from build123d import *

# Parameters (mm, degrees)
SKETCH1_W             = 60.96
SKETCH1_H             = 73.66
BOSS_EXTRUDE1_DEPTH   = 3.0734
FILLET1_R             = 2.54
F_8_CLEARANCE_HOLE1_D = 4.4958


with BuildPart() as part:
    # Sketch1 → Boss-Extrude1 (new body)
    with BuildSketch(Plane(origin=(0, 0, 0), x_dir=(1, 0, 0), z_dir=(0, 1, 0))):
        with Locations((30.48, 36.83)):
            Rectangle(SKETCH1_W, SKETCH1_H)
    extrude(amount=BOSS_EXTRUDE1_DEPTH)

    # Fillet1
    fillet1_edges = [part.edges().sort_by_distance(p)[0] for p in [
        (0, 1.5367, -73.66),
        (60.96, 1.5367, -73.66),
        (60.96, 1.5367, 0),
        (0, 1.5367, 0),
    ]]
    fillet(fillet1_edges, radius=FILLET1_R)

    # #8 Clearance Hole1 (through all)
    with Locations(Plane(origin=(0, 3.0734, 0), x_dir=(1, 0, 0), z_dir=(0, 1, 0))):
        with Locations((54.356, 67.056), (54.356, 6.604), (6.604, 67.056), (6.604, 6.604)):
            Hole(F_8_CLEARANCE_HOLE1_D / 2)


solid = part.part
Can you work these out from the model? Positions are in its coordinate system, mm. Coordinates: 2 decimals unless noted, no trailing zeros. Order: outer loops, then holes, each group sorted by start corner. A loop starts at its lowest first (then second) coordinate and runs counter-clockwise, first axis right, second up. Notation, with made-up numbers: M 1,88 L 15,88 A17 ccw 15,111 Z; hole C 46,44.5 d10. An arc over 180 degrees is marked long. Answer as CSV lines item,"result".
(1) I'm going to push flat-ended pins straight in: pin 1 (4 mm diameter, centred on x = 6.604, z = -6.604, fed in from -Y); pin 2 (5 mm diameter, centred on x = 54.356, z = -67.056, fed in from +Y). Where does each tip first touch, or does it pass through?
Geometry check:
pin 1,"through"
pin 2,"y = 3.07"
(2) Please list where these lines run through material, in increasing order: L1, parallel to X at y = 1.6, z = -67.5; L2, parallel to X at y = 1.55, z = -8.5.
Geometry check:
L1,"0 to 4.4, 8.81 to 52.15, 56.56 to 60.96"
L2,"0 to 5.4, 7.81 to 53.15, 55.56 to 60.96"
(3) Suppose I cut it at B-B on z = -8. Please give me the cut outline in (x, y), plus the area to 3 significant figures.
Geometry check:
outline,"M 0,0 L 4.84,0 L 4.84,3.07 L 0,3.07 Z; M 8.37,0 L 52.59,0 L 52.59,3.07 L 8.37,3.07 Z; M 56.12,0 L 60.96,0 L 60.96,3.07 L 56.12,3.07 Z"
area,"166 mm^2"
(4) If we mould it in two halves opening along Z, with no side actions, what happens to faces 1 (the cylindrical face through (56.6, 1.5, -6.7)), 2 (the flat face through (30, 2, 0)), 3 (the cylindrical face through (60.236, 1.558, -72.896)), 4 (the flat face through (30, 3.073, -37))? For each: released by +Z, released by -Z, zero draft, split by the parting line, or undercut.
Geometry check:
face 1,"undercut"
face 2,"released by +Z"
face 3,"released by -Z"
face 4,"zero draft"
(5) Suppose I cut it at C-C on y = 1. Please give me the cut outline in (x, z).
Geometry check:
outline,"M 0,-71.12 A2.54 ccw 2.54,-73.66 L 58.42,-73.66 A2.54 ccw 60.96,-71.12 L 60.96,-2.54 A2.54 ccw 58.42,0 L 2.54,0 A2.54 ccw 0,-2.54 Z; hole C 6.6,-67.06 d4.5; hole C 6.6,-6.6 d4.5; hole C 54.36,-67.06 d4.5; hole C 54.36,-6.6 d4.5"
(6) Suppose I cut it at A-A on x = 7.5. Please give me the cut outline in (y, z), plus the area to 3 significant figures.
Geometry check:
outline,"M 0,-73.66 L 3.07,-73.66 L 3.07,-69.12 L 0,-69.12 Z; M 0,-64.99 L 3.07,-64.99 L 3.07,-8.67 L 0,-8.67 Z; M 0,-4.54 L 3.07,-4.54 L 3.07,0 L 0,0 Z"
area,"201 mm^2"
